Could you check a few things on this model? Use its own coordinates, in mm. A direction names the side the tool comes from. Round coordinates to 2 decimals unless told otherwise and drop trailing zeros. Loops run counter-clockwise (first coordinate to the right, second up) from the corner with the lowest first, then second, coordinate; pieces in that order, holes last. Notation, with made-up numbers: M 60.5,85.25 L 113.5,85.25 A5 ccw 113.5,90.25 Z; hole C -33,-16 d3. An arc over 180 degrees is marked long. One line per item, written item: value. Start each with the question number.
Q1. Imagine slicing it at A-A (x = 15.7). Please give me the cut outline in (y, z).
Q2. Thinking about a two-plate mould opening in X: for faces 1 (the face through (12, 1, 6)), 2 (the face through (-22.8, 3, -1)), 3 (the face through (-14.27, -3.55, -0.74)), which applies, released by +X, released by -X, zero draft, split by the parting line, or undercut?
Q3. Please list where these lines run through material, in increasing order: line 1 along Y through (x, z) = (-15.7, -0.5); line 2 along Z through (x, y) = (5.5, -0.5); line 3 along Y through (x, z) = (-6, 2.75).
Q4. Imagine slicing it at C-C (z = 0.75). Please give me the cut outline in (x, y), then the cut area to 3 significant figures.
Q5. I'm going to push flat-ended pins straight in: pin 1 Ø2.5 at (x, y) = (15.7, -4) entering from -Z; pin 2 Ø3 at (y, z) = (1, 2.5) entering from -X; pin 3 Ø2 at (y, z) = (0.5, 1.5) entering from +X; pin 4 Ø1.2 at (x, z) = (12.5, 2.5) entering from +Y. Where does each tip first touch, or does it pass through?
Q6. Imagine slicing it at D-D (y = -4.5). Please give me the cut outline in (x, z).
Q7. Which directions (+Z, -Z, +X, -X, +Y, -Y) give clear straight access to the entire face, cutting with the end or side of a thin tool? Please do faces 4 (the face through (9, 1, 2)), 5 (the face through (4, -2, 2)), 6 (the face through (4, 4, 2)), 7 (the face through (5.57, 1.65, 4.99)), 8 (the face through (-15, 1, 2)).
Q8. Imagine slicing it at B-B (z = -1). Please give me the cut outline in (x, y).
Autodesk Fusion 360 part; units mm, degrees
sketch "Sketch1" plane through (0, 0, 0) normal (0, 0, 1) x (1, 0, 0)
  line L0 (-22.8, 10) -> (22.8, 10)
  line L1 (22.8, 10) -> (22.8, -10)
  line L2 (22.8, -10) -> (-22.8, -10)
  line L3 (-22.8, -10) -> (-22.8, 10)
  line L4 (-22.8, 10) -> (22.8, -10) construction
  line L5 (-15, 4) -> (-9, 4)
  line L6 (-9, 4) -> (-9, -2)
  line L7 (-9, -2) -> (-15, -2)
  line L8 (-15, -2) -> (-15, 4)
  line L9 (0, 10) -> (0, -10) construction
  line L10 (-1, -2) -> (-7, -2)
  line L11 (-7, -2) -> (-7, 4)
  line L12 (-7, 4) -> (-1, 4)
  line L13 (-1, 4) -> (-1, -2)
  line L14 (7, 4) -> (1, 4)
  line L15 (1, 4) -> (1, -2)
  line L16 (1, -2) -> (7, -2)
  line L17 (7, -2) -> (7, 4)
  line L18 (15, 4) -> (9, 4)
  line L19 (9, 4) -> (9, -2)
  line L20 (15, -2) -> (15, 4)
  line L21 (9, -2) -> (15, -2)
  circle A0 centre (-15.7, -4) radius 1.5
  circle A1 centre (15.7, -4) radius 1.5
  line L22 (-15.7, -4) -> (15.7, -4) construction
  dimension "d1" = 45.6
  dimension "d2" = 20
  dimension "d3" = 6
  dimension "d4" = 6
  dimension "d5" = 2
  dimension "d6" = 1
  dimension "d7" = 6
  dimension "d33" = 7.1
  dimension "d34" = 3
  dimension "d37" = 3
  dimension "d38" = 6
  dimension "d59" = 7.1
extrude "Extrude7" add sketch "Sketch1" against normal blind 1.5 contours L0 L1 L2 L3 | L5 L6 L7 L8 | L10 L11 L12 L13 | L14 L15 L16 L17 | L18 L19 L20 L21
extrude "Extrude8" add sketch "Sketch1" along normal blind 4 contours L5 L6 L7 L8 | L10 L11 L12 L13 | L14 L15 L16 L17 | L18 L19 L20 L21
sketch "Sketch6" plane through (0, 0, 4) normal (0, 0, 1) x (-1, 0, 0)
  line L0 (15, 2) -> (9, 2)
  line L1 (9, 2) -> (9, -4)
  line L2 (9, -4) -> (15, -4)
  line L3 (15, -4) -> (15, 2)
  line L4 (15, -4) -> (9, 2) construction
  circle A0 centre (12, -1) radius 1.7
  dimension "d44" = 3.4
sketch "Sketch7" plane through (0, 0, 4) normal (0, 0, 1) x (-1, 0, 0)
  line L0 (1, -4) -> (7, -4)
  line L1 (7, -4) -> (7, 2)
  line L2 (7, 2) -> (1, 2)
  line L3 (1, 2) -> (1, -4)
  line L4 (7, -4) -> (1, 2) construction
  circle A0 centre (4, -1) radius 1.7
  dimension "d45" = 3.4
extrude "Extrude9" add sketch "Sketch6" sketch "Sketch7" along normal blind 2 contours A0 of sketch 2 contours A0
mirror "Mirror2" about plane through (0, 0, 0) normal (1, 0, 0) of "Extrude9"
sketch "Sketch8" plane through (0, 0, 0) normal (0, 0, 1) x (-1, 0, 0)
  line L0 (-9, 2) -> (-9, -4)
  line L1 (-9, -4) -> (-15, -4)
  line L2 (-15, -4) -> (-15, 2)
  line L3 (-15, 2) -> (-9, 2)
  line L4 (15, 2) -> (15, -4)
  line L5 (15, -4) -> (9, -4)
  line L6 (9, -4) -> (9, 2)
  line L7 (9, 2) -> (15, 2)
  line L8 (-7, 2) -> (-1, 2)
  line L9 (-1, 2) -> (-1, -4)
  line L10 (-1, -4) -> (-7, -4)
  line L11 (-7, -4) -> (-7, 2)
  line L12 (1, -4) -> (1, 2)
  line L13 (1, 2) -> (7, 2)
  line L14 (7, 2) -> (7, -4)
  line L15 (7, -4) -> (1, -4)
  circle A0 centre (15.7, 4) radius 1.5
  circle A1 centre (-15.7, 4) radius 1.5
  line L16 (22.8, 10) -> (-22.8, 10)
  line L17 (-22.8, 10) -> (-22.8, -10)
  line L18 (-22.8, -10) -> (22.8, -10)
  line L19 (22.8, -10) -> (22.8, 10)
  line L20 (16.3985, 10) -> (22.8, 3.5985)
  line L21 (15.7, 4) -> (19.5993, 6.7993) construction
  line L22 (0, 0) -> (0, -10) construction
  line L23 (-16.3985, 10) -> (-22.8, 3.5985)
  dimension "d51" = 45
  dimension "d52" = 4.8
extrude "Extrude10" cut sketch "Sketch8" against normal blind 1.5 contours L16 L19 L20 | L16 L17 L23
move_face "OffsetFaces1" offset -2 1 faces at (5.4662, -10, -0.5)
extrude "Extrude1" [suppressed]
extrude "Extrude2" [suppressed]
sketch "Sketch2" plane through (0, 0, 4) normal (0, 0, 1) x (-1, 0, 0)
  line L0 (15, 2) -> (9, 2)
  line L1 (9, 2) -> (9, -4)
  line L2 (9, -4) -> (15, -4)
  line L3 (15, -4) -> (15, 2)
  circle A0 centre (12, -1) radius 2
  line L4 (15, -4) -> (9, 2) construction
  dimension "d12" = 4
extrude "Extrude3" [suppressed]
sketch "Sketch3" plane through (0, 0, 4) normal (0, 0, 1) x (-1, 0, 0)
  line L0 (1, -4) -> (7, -4)
  line L1 (7, -4) -> (7, 2)
  line L2 (7, 2) -> (1, 2)
  line L3 (1, 2) -> (1, -4)
  line L4 (7, -4) -> (1, 2) construction
  circle A0 centre (4, -1) radius 2
  dimension "d15" = 4
extrude "Extrude4" [suppressed]
mirror "Mirror1" [suppressed]
sketch "Sketch4" plane through (0, 0, 0) normal (0, 0, 1) x (-1, 0, 0)
  line L0 (-9, 2) -> (-9, -4)
  line L1 (-9, -4) -> (-15, -4)
  line L2 (-15, -4) -> (-15, 2)
  line L3 (-15, 2) -> (-9, 2)
  line L4 (15, 2) -> (15, -4)
  line L5 (15, -4) -> (9, -4)
  line L6 (9, -4) -> (9, 2)
  line L7 (9, 2) -> (15, 2)
  line L8 (-7, 2) -> (-1, 2)
  line L9 (-1, 2) -> (-1, -4)
  line L10 (-1, -4) -> (-7, -4)
  line L11 (-7, -4) -> (-7, 2)
  line L12 (1, -4) -> (1, 2)
  line L13 (1, 2) -> (7, 2)
  line L14 (7, 2) -> (7, -4)
  line L15 (7, -4) -> (1, -4)
  line L16 (22.8, 10) -> (-22.8, 10)
  line L17 (-22.8, 10) -> (-22.8, -10)
  line L18 (-22.8, -10) -> (22.8, -10)
  line L19 (22.8, -10) -> (22.8, 10)
  circle A0 centre (-19.6, -3.8) radius 1.5
  circle A1 centre (17.3, 3.5) radius 1.5
  dimension "d20" = 3
  dimension "d21" = 3.2
  dimension "d22" = 6.2
  dimension "d23" = 3
  dimension "d24" = 6.5
  dimension "d25" = 5.5
extrude "Extrude5" [suppressed]
sketch "Sketch5" plane through (0, 0, 0) normal (0, 0, 1) x (-1, 0, 0)
  circle A0 centre (-19.6, -3.8) radius 1.5
  circle A1 centre (17.3, 3.5) radius 1.5
  line L0 (-9, 2) -> (-9, -4)
  line L1 (-9, -4) -> (-15, -4)
  line L2 (-15, -4) -> (-15, 2)
  line L3 (-15, 2) -> (-9, 2)
  line L4 (15, 2) -> (15, -4)
  line L5 (15, -4) -> (9, -4)
  line L6 (9, -4) -> (9, 2)
  line L7 (9, 2) -> (15, 2)
  line L8 (-7, 2) -> (-1, 2)
  line L9 (-1, 2) -> (-1, -4)
  line L10 (-1, -4) -> (-7, -4)
  line L11 (-7, -4) -> (-7, 2)
  line L12 (1, -4) -> (1, 2)
  line L13 (1, 2) -> (7, 2)
  line L14 (7, 2) -> (7, -4)
  line L15 (7, -4) -> (1, -4)
  line L16 (22.8, 10) -> (-22.8, 10)
  line L17 (-22.8, 10) -> (-22.8, -10)
  line L18 (-22.8, -10) -> (22.8, -10)
  line L19 (22.8, -10) -> (22.8, 10)
  line L20 (14.3, 3.2) -> (-22.8, 3.2)
  line L21 (-22.8, 3.2) -> (-22.8, 10)
  line L22 (-22.8, 10) -> (14.3, 10)
  line L23 (14.3, 10) -> (14.3, 3.2)
  dimension "d28" = 6.8
  dimension "d29" = 8.5
extrude "Extrude6" [suppressed]
equation "d22 = 4.7 mm + 1.5 mm"
Report:
1. outline: M -8,-1.5 L -5.5,-1.5 L -5.5,0 L -8,0 Z; M -2.5,-1.5 L 10,-1.5 L 10,0 L -2.5,0 Z
2. face 1: zero draft
2. face 2: released by -X
2. face 3: undercut
3. line 1: y = -8 to -5.5, -2.5 to 10
3. line 2: z = -1.5 to 4
3. line 3: y = -2 to 4
4. outline: M -15,-2 L -9,-2 L -9,4 L -15,4 Z; M -7,-2 L -1,-2 L -1,4 L -7,4 Z; M 1,-2 L 7,-2 L 7,4 L 1,4 Z; M 9,-2 L 15,-2 L 15,4 L 9,4 Z
4. area: 144 mm²
5. pin 1: passes through
5. pin 2: stops at x = -15
5. pin 3: stops at x = 15
5. pin 4: stops at y = 4
6. outline: M -21.9,-1.5 L -17.11,-1.5 L -17.11,0 L -21.9,0 Z; M -14.29,-1.5 L 14.29,-1.5 L 14.29,0 L -14.29,0 Z; M 17.11,-1.5 L 21.9,-1.5 L 21.9,0 L 17.11,0 Z
7. face 4: +Z, +Y, -Y
7. face 5: +Z, +X, -X, -Y
7. face 6: +Z, +X, -X, +Y
7. face 7: +Z
7. face 8: +Z, -X, +Y, -Y
8. outline: M -22.8,-3.6 L -18.4,-8 L 18.4,-8 L 22.8,-3.6 L 22.8,10 L -22.8,10 Z; hole C -15.7,-4 d3; hole C 15.7,-4 d3
